Design review of the part built by this model. Coordinates are the model's own, in mm. Give positions to 0.01 mm unless a question says otherwise; leave off trailing zeros. Order: outer loops, then holes, each group sorted by start corner. A loop starts at its lowest first (then second) coordinate and runs counter-clockwise, first axis right, second up. Notation, with made-up numbers: (43.25, 47) -> (80.25, 47) arc R26 ccw to (80.25, 76) -> close; hole circle Ø2 at (-12.5, -39.75). An arc over 180 degrees is marked (long way). One line per item, written item: value.
from build123d import *

# Parameters (mm, degrees)
SKETCH1_W           = 20
SKETCH1_H           = 35
BOSS_EXTRUDE1_DEPTH = 12.6
CUT_EXTRUDE1_REACH  = 14.6
SKETCH2_R           = 1.5


with BuildPart() as part:
    # Sketch1 → Boss-Extrude1 (new body)
    with BuildSketch(Plane(origin=(0, 0, 0), x_dir=(1, 0, 0), z_dir=(0, 1, 0))):
        Rectangle(SKETCH1_W, SKETCH1_H)
    extrude(amount=BOSS_EXTRUDE1_DEPTH)

    # Sketch2 → Cut-Extrude1 (cut, up to next)
    with BuildSketch(Plane.XZ, mode=Mode.PRIVATE) as cut_extrude1_sk1:
        with Locations((-5.990644946, 12.563355097)):
            Circle(SKETCH2_R)
    cut_extrude1_tool1 = extrude(cut_extrude1_sk1.sketch, amount=-CUT_EXTRUDE1_REACH, mode=Mode.PRIVATE) & part.part
    add(cut_extrude1_tool1.solids().sort_by_distance((-5.990645, 0, 12.563355))[0], mode=Mode.SUBTRACT)
    # Sketch2 → Cut-Extrude1 (cut, up to next)
    with BuildSketch(Plane.XZ, mode=Mode.PRIVATE) as cut_extrude1_sk2:
        with Locations((4.609355054, -10.036644903)):
            Circle(SKETCH2_R)
    cut_extrude1_tool2 = extrude(cut_extrude1_sk2.sketch, amount=-CUT_EXTRUDE1_REACH, mode=Mode.PRIVATE) & part.part
    add(cut_extrude1_tool2.solids().sort_by_distance((4.609355, 0, -10.036645))[0], mode=Mode.SUBTRACT)


solid = part.part
Item 1: Clearance check with a flat-ended pin moving along its axis: P1, Ø2.5, axis at x = -5.99, z = 12.56, coming from the +Y side (3 decimals). State where the tip first meets the part, or that it passes through.
Returned:
P1: through
Item 2: To check wall thickness, follow line 1 along X through (y, z) = (5.75, 13.5); line 2 along Z through (x, y) = (4, 0.5); line 3 along X through (y, z) = (4.5, 13). State the ranges of each line that lie inside material, in increasing order. Write a range as from..to.
Returned:
line 1: -10..-7.16, -4.82..10
line 2: -17.5..-11.41, -8.67..17.5
line 3: -10..-7.43, -4.56..10
Item 3: Add section A-A on y = 10.25. Give the boundary of the cut face in (x, z).
Returned:
outline: (-10, -17.5) -> (10, -17.5) -> (10, 17.5) -> (-10, 17.5) -> close; hole circle Ø3 at (-5.99, 12.56); hole circle Ø3 at (4.61, -10.04)
Item 4: Draft analysis for pull direction Z (two halves, no side actions). For faces 1 (the flat face through (0, 12.6, 0)), 2 (the cylindrical face through (-4.6, 6.2, 12)), 3 (the flat face through (0, 6, -17.5)), state which applies: pulls with the +Z half, pulls with the -Z half, needs draft (parallel to the pull), parting line crosses it, or undercut.
Returned:
face 1: needs draft
face 2: undercut
face 3: pulls with the -Z half
